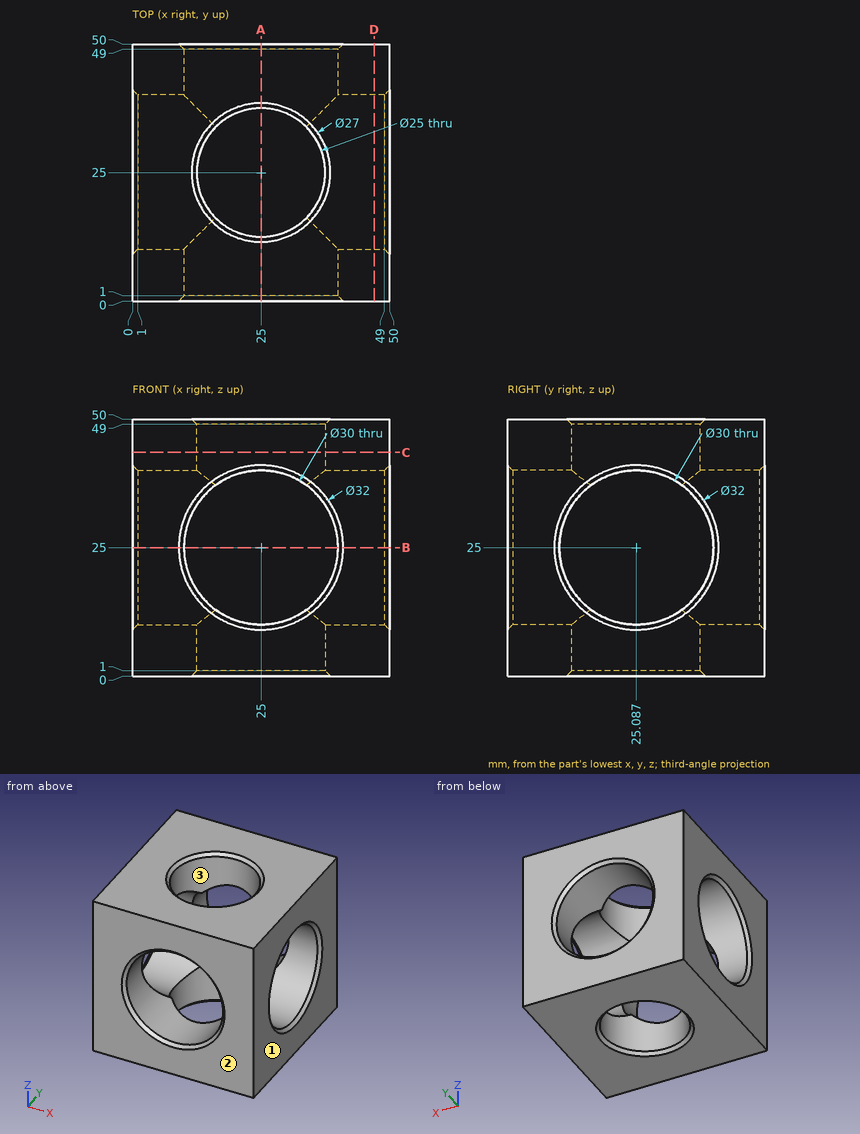
Input: dimensioned drawing with shaded views. Units: mm. Origin: part minimum x, y, z. Coordinates: 2 decimals unless noted, no trailing zeros. Write each loop counter-clockwise with the first axis right and the second up, starting at its lowest first coordinate (ties: lowest second). Pieces come first, ordered by that corner, then holes. Notation, with made-up numbers: M -29.5,62 L -12.5,62 A14 cw -12.5,84 Z; hole C 11.25,-36 d9. An arc over 180 degrees is marked long. Answer as a JSON object with one key per item and string values. Group by question number.
(1) Ray query, line 1 along Z through (x, y) = (25, 4); line 2 along X through (y, z) = (25, 42). Return the intervals inside material, ascending. Write a range as [from, to].
(2) Section C-C on z = 43.5. Output: boundary loops of the cut face in (x, y).
(3) Section B-B on z = 25. Output: boundary loops of the cut face in (x, y).
(4) Mould query, pull axis X, two halves, no side actions, for the marked faces 1, 2 and 3. Classes: pulls with the +X half, pulls with the -X half, needs draft (parallel to the pull), parting line crosses it, or undercut.
(5) Section A-A on x = 25. Output: boundary loops of the cut face in (y, z).
(6) Section D-D on x = 47. Output: boundary loops of the cut face in (y, z).
(7) Contact query for flat-ended pins moving along their axis: P1, Ø12, axis at x = 32, y = 22.5, coming from the -Z side; P2, Ø6, axis at x = 37.5, z = 24, coming from the +Y side. Output: stop coordinate, or through.
Result set:
{
 "1": {"line 1": "z = [0, 10], [40, 50]", "line 2": "x = [0, 12.5], [37.5, 50]"},
 "2": {"outline": "M 0,0 L 50,0 L 50,50 L 0,50 Z; hole C 25,25 d25"},
 "3": {"outline": "M 0,0 L 9,0 L 10,1 L 10,10.09 L 1,10.09 L 0,9.09 Z; M 0,41.09 L 1,40.09 L 10,40.09 L 10,49 L 9,50 L 0,50 Z; M 40,1 L 41,0 L 50,0 L 50,9.09 L 49,10.09 L 40,10.09 Z; M 40,40.09 L 49,40.09 L 50,41.09 L 50,50 L 41,50 L 40,49 Z"},
 "4": {"face 1": "pulls with the +X half", "face 2": "needs draft", "face 3": "undercut"},
 "5": {"outline": "M 0,0 L 11.5,0 L 12.5,1 L 12.5,10 L 1,10 L 0,9 Z; M 0,41 L 1,40 L 12.5,40 L 12.5,49 L 11.5,50 L 0,50 Z; M 37.5,1 L 38.5,0 L 50,0 L 50,9 L 49,10 L 37.5,10 Z; M 37.5,40 L 49,40 L 50,41 L 50,50 L 38.5,50 L 37.5,49 Z"},
 "6": {"outline": "M 0,0 L 50,0 L 50,50 L 0,50 Z; hole C 25.09,25 d30"},
 "7": {"P1": "stops at z = 0.07", "P2": "stops at y = 49.54"}
}
